Build history of the part. All positions in model axes, mm. Face numbers are marked on the shaded views. A direction names the side the tool comes from. Round coordinates to 2 decimals unless told otherwise and drop trailing zeros. Order: outer loops, then holes, each group sorted by start corner. A loop starts at its lowest first (then second) coordinate and runs counter-clockwise, first axis right, second up. Notation, with made-up numbers: (81, -27.75) -> (88, -27.75) arc R30 cw to (88, -5.75) -> close; hole circle Ø9 at (23, 45.5). An arc over 180 degrees is marked (long way). Write item = value, one per line.
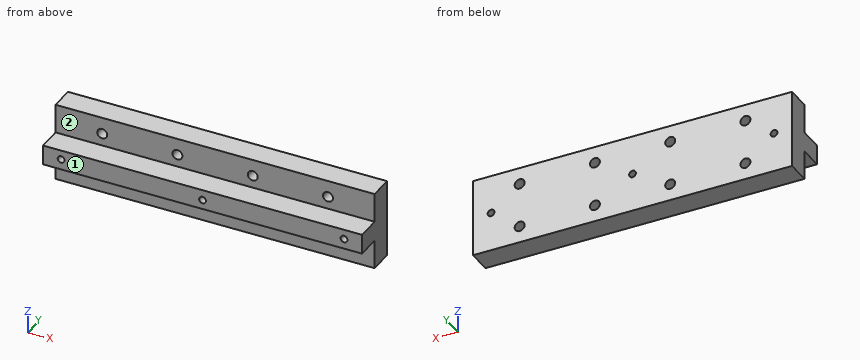
from build123d import *

# Parameters (mm, degrees)
SKETCH4_W                       = 106
SKETCH4_H                       = 16
BOSS_EXTRUDE2_DEPTH             = 13
CUT_EXTRUDE3_START              = -9.7
SKETCH25_W                      = 106
SKETCH25_H                      = 8.1
CUT_EXTRUDE3_DEPTH              = 107.216438698
M4X0_7_TAPPED_HOLE1_D           = 3.3
MIRROR1_START                   = -24.601316976
MIRROR1_OUTLINE_W               = 106
MIRROR1_OUTLINE_H               = 13
MIRROR1_OUTLINE_R               = 1.65
MIRROR1_DEPTH                   = 7.951316976
MIRROR1_START_2                 = -32.65
MIRROR1_2_OUTLINE_W             = 106
MIRROR1_2_OUTLINE_H             = 3.3
MIRROR1_2_DEPTH                 = 8.048683024
F_4_40_TAPPED_HOLE1_D           = 2.2606
F_4_40_TAPPED_HOLE1_ON_FACE_2_D = 2.2606


# Read off the part's stored shape, not the designer's step: Mirror1
with BuildPart() as part:
    # Sketch4 → Boss-Extrude2 (new body)
    with BuildSketch(Plane.XY):
        with Locations((-36.891047602, -24.65)):
            Rectangle(SKETCH4_W, SKETCH4_H)
    extrude(amount=-BOSS_EXTRUDE2_DEPTH)

    # Sketch25 → Cut-Extrude3 (cut)
    with BuildSketch(Plane.XY.offset(CUT_EXTRUDE3_START)):
        with Locations((-36.891047602, -28.651316976)):
            Rectangle(SKETCH25_W, SKETCH25_H)
    extrude(amount=CUT_EXTRUDE3_DEPTH, mode=Mode.SUBTRACT)

    # M4x0.7 Tapped Hole1 (through all)
    with Locations(Plane(origin=(-74.391047602, -16.65, -5.55), x_dir=(0, 0, 1), z_dir=(0, 1, 0))):
        with Locations((0, 0), (0, 25), (0, 75), (0, 50)):
            Hole(M4X0_7_TAPPED_HOLE1_D / 2)

    # Mirror1 outline → Mirror1 (add)
    with BuildSketch(Plane(origin=(0, 0, 0), x_dir=(1, 0, 0), z_dir=(0, 1, 0)).offset(MIRROR1_START)):
        with Locations((-36.891047602, 19.5)):
            Rectangle(MIRROR1_OUTLINE_W, MIRROR1_OUTLINE_H)
        with Locations((-74.391047602, 20.45)):
            Circle(MIRROR1_OUTLINE_R, mode=Mode.SUBTRACT)
        with Locations((-49.391047602, 20.45)):
            Circle(MIRROR1_OUTLINE_R, mode=Mode.SUBTRACT)
        with Locations((-24.391047602, 20.45)):
            Circle(MIRROR1_OUTLINE_R, mode=Mode.SUBTRACT)
        with Locations((0.608952398, 20.45)):
            Circle(MIRROR1_OUTLINE_R, mode=Mode.SUBTRACT)
    extrude(amount=MIRROR1_DEPTH)

    # Mirror1 2 outline → Mirror1 2 (add)
    with BuildSketch(Plane(origin=(0, 0, 0), x_dir=(1, 0, 0), z_dir=(0, 1, 0)).offset(MIRROR1_START_2)):
        with Locations((-36.891047602, 14.65)):
            Rectangle(MIRROR1_2_OUTLINE_W, MIRROR1_2_OUTLINE_H)
    extrude(amount=MIRROR1_2_DEPTH)

    # #4-40 Tapped Hole1 (through all)
    with Locations(Plane(origin=(-83.891047602, -32.65, -12.801414568), x_dir=(0, 0, -1), z_dir=(0, -1, 0))):
        with Locations((0, 0), (0.13677014, 94), (0.355392609, 47)):
            Hole(F_4_40_TAPPED_HOLE1_D / 2)

    # #4-40 Tapped Hole1 on face 2 (through all)
    with Locations(Plane(origin=(-13.707536503, 0, 46.33240541), x_dir=(0, 0, -1), z_dir=(0, -1, 0))):
        with Locations((0, 0)):
            Hole(F_4_40_TAPPED_HOLE1_ON_FACE_2_D / 2)


solid = part.part
Q1. Probe probe 1 along X at (y, z) = (-21.25, -20.45); probe 2 along X at (y, z) = (-19, -13); probe 3 along Z at (x, y) = (10, -28.75). List the from-to ranges inside material, lowest first.
Check values:
probe_1 = -89.89 to -76.04, -72.74 to -51.04, -47.74 to -26.04, -22.74 to -1.04, 2.26 to 16.11
probe_2 = -89.89 to -85, -82.78 to -38.01, -35.77 to 8.98, 11.24 to 16.11
probe_3 = -16.3 to -14.06, -11.81 to -9.7
Q2. Which spindle directions (+Z, -Z, +X, -X, +Y, -Y) get a long thin tool onto all of the face, cutting with end or side? Do the marked faces 1 and 2. Say none if no direction does.
Check values:
face_1 = +Z, -Z, +X, -X, -Y
face_2 = +Z, +X, -X, -Y
Q3. Cut at D-D, the plane y = -26.25. List the corners of the cut face in (x, z).
Check values:
outline = (-89.89, -16.3) -> (16.11, -16.3) -> (16.11, -9.7) -> (-89.89, -9.7) -> close; hole circle Ø2.26 at (-83.89, -12.8); hole circle Ø2.26 at (-36.89, -13.16); hole circle Ø2.26 at (10.11, -12.94)
Q4. Cut at A-A, the plane z = -20.45. List the corners of the cut face in (x, y).
Check values:
outline = (-89.89, -24.6) -> (-76.04, -24.6) -> (-76.04, -16.65) -> (-89.89, -16.65) -> close; (-72.74, -24.6) -> (-51.04, -24.6) -> (-51.04, -16.65) -> (-72.74, -16.65) -> close; (-47.74, -24.6) -> (-26.04, -24.6) -> (-26.04, -16.65) -> (-47.74, -16.65) -> close; (-22.74, -24.6) -> (-1.04, -24.6) -> (-1.04, -16.65) -> (-22.74, -16.65) -> close; (2.26, -24.6) -> (16.11, -24.6) -> (16.11, -16.65) -> (2.26, -16.65) -> close
Q5. Cut at B-B, the plane x = -7.5. List the corners of the cut face in (y, z), and give its area (3 significant figures).
Check values:
outline = (-32.65, -16.3) -> (-24.6, -16.3) -> (-24.6, -26) -> (-16.65, -26) -> (-16.65, 0) -> (-24.6, 0) -> (-24.6, -9.7) -> (-32.65, -9.7) -> close
area = 260 mm²
Q6. Cut at C-C, the plane y = -22. Give the number of separate pieces and of enclosed holes in the cut face, and give its area (3 significant figures).
Check values:
separate_pieces = 1
enclosed_holes = 11
area = 2,680 mm²
Q7. Flat gauge pins, fed straight in: pin 1 (4 mm diameter, centred on x = -20, y = -28.5, fed in from -Z); pin 2 (3 mm diameter, centred on x = -24.39, z = -20.45, fed in from -Y); pin 3 (5.5 mm diameter, centred on x = 0.61, z = -5.55, fed in from -Y); pin 4 (4 mm diameter, centred on x = -31, y = -30, fed in from +Z). Where does each tip first touch, or does it go through?
Check values:
pin_1 = -16.3
pin_2 = through
pin_3 = -24.6
pin_4 = -9.7
